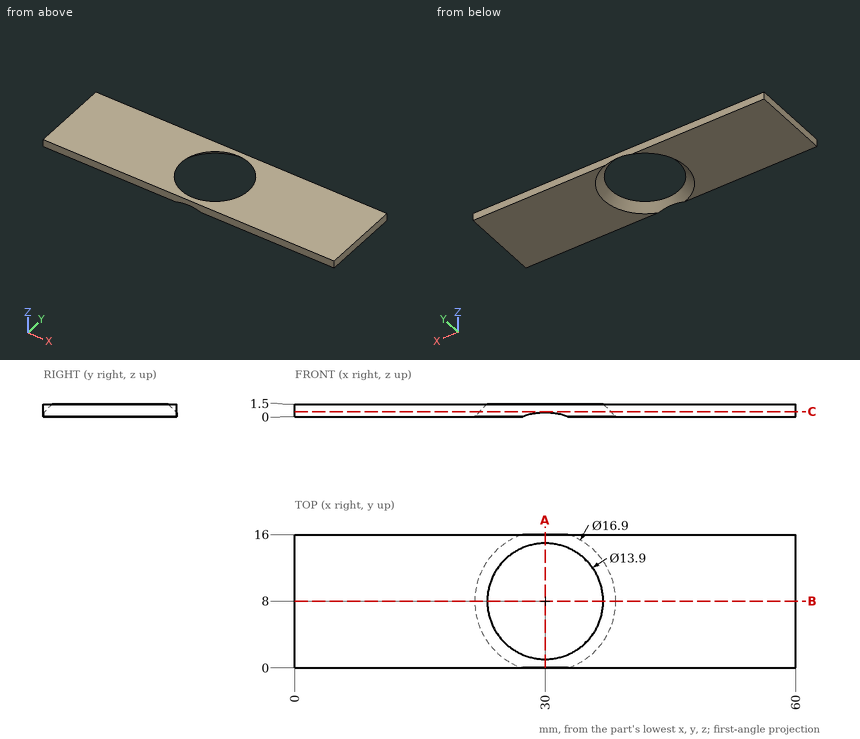
Geometry: see drawing. Coordinates: mm, zero at the bounding-box minimum. Round coordinates to 2 decimals unless told otherwise and drop trailing zeros. Loops run counter-clockwise (first coordinate to the right, second up) from the corner with the lowest first, then second, coordinate; pieces in that order, holes last. Notation, with made-up numbers: M 12,74 L 55,74 A28 ccw 55,95 Z; hole C 41,-20.5 d1. An arc over 180 degrees is marked long. Use a Markdown table: item, result. Add a question column.
1. Section query C-C on z = 0.6. Return the cut outline in (x, y).
2. Section query A-A on x = 30. Return the cut outline in (y, z).
3. Line query: line 1 (X direction, y = 10.25, z = 1.15); line 2 (X direction, y = 12.25, z = 1.15); line 3 (Y direction, x = 31, z = 0.7). Output: solid intervals per line, ascending.
4. Section query B-B on y = 8. Return the cut outline in (x, z), then the cut area to 3 significant figures.
5. Contact query for a flat-ended pin moving along its axis: P1, Ø3, axis at x = 35, y = 13, coming from the -Z side. Output: stop coordinate, or through.
Reported:
| question | item | result |
|---|---|---|
| 1 | outline | M 0,0 L 60,0 L 60,16 L 0,16 Z; hole C 30,8 d15.7 |
| 2 | outline | M 0,0.45 L 1.05,1.5 L 0,1.5 Z; M 14.95,1.5 L 16,0.45 L 16,1.5 Z |
| 3 | line 1 | x = 0 to 23.06, 36.94 to 60 |
| 3 | line 2 | x = 0 to 24.06, 35.94 to 60 |
| 3 | line 3 | y = 0 to 0.31, 15.69 to 16 |
| 4 | outline | M 0,0 L 21.55,0 L 23.05,1.5 L 0,1.5 Z; M 36.95,1.5 L 38.45,0 L 60,0 L 60,1.5 Z |
| 4 | area | 66.9 mm² |
| 5 | P1 | stops at z = 0 |
